Here's how the part is built. I have some questions about the finished solid (model axes, mm). Face numbers are marked on the shaded views. Round coordinates to 2 decimals unless told otherwise and drop trailing zeros. Loops run counter-clockwise (first coordinate to the right, second up) from the corner with the lowest first, then second, coordinate; pieces in that order, holes last. Notation, with made-up numbers: (82, -37.75) -> (141, -37.75) arc R19 cw to (141, -33.75) -> close; hole circle Ø1 at (55.5, 60.5). An arc over 180 degrees is marked (long way). One line per item, written item: value. Start each with the question number.
```python
from build123d import *

# Parameters (mm, degrees)
F0_W           = 30
F0_H           = 50
F1_DEPTH       = 6
F3_D           = 4.4
F3_CSINK_D     = 8.96
F3_CSINK_ANGLE = 90
F4_W           = 10
F4_H           = 50
F5_DEPTH       = 3.5
F6_R           = 2.5


with BuildPart() as f1:
    # F0 (on Top) → F1 (new body)
    with BuildSketch(Plane.XY):
        Rectangle(F0_W, F0_H)
    extrude(amount=F1_DEPTH)

    # F3 (through all)
    with Locations(Plane.XY.offset(6)):
        with Locations((5, 15), (5, -15)):
            CounterSinkHole(F3_D / 2, F3_CSINK_D / 2, counter_sink_angle=F3_CSINK_ANGLE)

    # F4 (on face) → F5 (cut)
    with BuildSketch(Plane(origin=(0, 0, 0), x_dir=(1, 0, 0), z_dir=(0, 0, -1))):
        with Locations((-10, 0)):
            Rectangle(F4_W, F4_H)
    extrude(amount=-F5_DEPTH, mode=Mode.SUBTRACT)

    # F6
    f6_edges = [f1.edges().sort_by_distance(p)[0] for p in [
        (-15, -25, 4.75),
        (15, -25, 3),
        (-15, 25, 4.75),
        (15, 25, 3),
    ]]
    fillet(f6_edges, radius=F6_R)


solid = f1.part
```
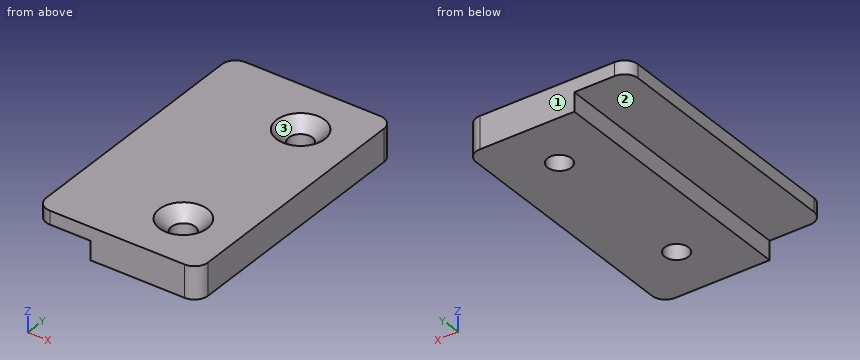
Q1. I want a section at B-B on x = 5. Please give me the cut outline in (y, z), plus the area to 3 significant figures.
Q2. I want a section at D-D on z = 1.25. Please give me the cut outline in (x, y).
Q3. I want a section at C-C on y = -15. Please give me the cut outline in (x, z), plus the area to 3 significant figures.
Q4. If I drill on line 1 along Y through (x, z) = (5, 1.25); line 2 along X through (y, z) = (-15, 2.5); line 3 along Y through (x, z) = (3, 1.7), over which ranges is the centre line in solid material (lowest first)?
Q5. If we mould it in two halves opening along Y, with no side actions, what happens to the marked faces 1, 2 and 3? For each: released by +Y, released by -Y, zero draft, split by the parting line, or undercut.
Q6. Will this pin go through, and if not, where does the flat tip stop? P1, Ø1, axis at x = 2.5, y = 16, coming from the +Z side.
Q7. I want a section at A-A on z = 5.2. Please give me the cut outline in (x, y).
Answers below:
1. outline: (-25, 0) -> (-17.2, 0) -> (-17.2, 3.72) -> (-19.48, 6) -> (-25, 6) -> close; (-12.8, 0) -> (12.8, 0) -> (12.8, 3.72) -> (10.52, 6) -> (-10.52, 6) -> (-12.8, 3.72) -> close; (17.2, 0) -> (25, 0) -> (25, 6) -> (19.48, 6) -> (17.2, 3.72) -> close
1. area: 237 mm^2
2. outline: (-5, -25) -> (12.5, -25) arc R2.5 ccw to (15, -22.5) -> (15, 22.5) arc R2.5 ccw to (12.5, 25) -> (-5, 25) -> close; hole circle Ø4.4 at (5, -15); hole circle Ø4.4 at (5, 15)
3. outline: (-15, 3.5) -> (-5, 3.5) -> (-5, 0) -> (2.8, 0) -> (2.8, 3.72) -> (0.52, 6) -> (-15, 6) -> close; (7.2, 0) -> (15, 0) -> (15, 6) -> (9.48, 6) -> (7.2, 3.72) -> close
3. area: 113 mm^2
4. line 1: y = -25 to -17.2, -12.8 to 12.8, 17.2 to 25
4. line 2: x = -5 to 2.8, 7.2 to 15
4. line 3: y = -25 to -15.92, -14.08 to 14.08, 15.92 to 25
5. face 1: released by +Y
5. face 2: zero draft
5. face 3: undercut
6. P1: stops at z = 4.71
7. outline: (-15, -22.5) arc R2.5 ccw to (-12.5, -25) -> (12.5, -25) arc R2.5 ccw to (15, -22.5) -> (15, 22.5) arc R2.5 ccw to (12.5, 25) -> (-12.5, 25) arc R2.5 ccw to (-15, 22.5) -> close; hole circle Ø7.36 at (5, -15); hole circle Ø7.36 at (5, 15)
